```python
from build123d import *

# Parameters (mm, degrees)
F0_W      = 16
F0_H      = 16
F1_DEPTH  = 16
F2_R      = 2
F3_R      = 1.75
F4_DEPTH  = 1
F8_R      = 1.75
F8_R_2    = 1.7502183246
F9_DEPTH  = 1
F11_R     = 1.75
F12_DEPTH = 1
F14_R     = 1.75
F15_DEPTH = 1
F17_R     = 1.75
F18_DEPTH = 1
F20_R     = 1.75
F21_DEPTH = 1


# Not quite as in the source:
# - a fillet or chamfer that OpenCascade refuses, or shapes differently, is made with other operations: its cross-section is extruded or revolved along the edge and cut away or added


with BuildPart() as f1:
    # F0 (on Top) → F1 (new body)
    with BuildSketch(Plane.XY):
        Rectangle(F0_W, F0_H)
    extrude(amount=-F1_DEPTH)

    # F2
    f2_edges = [f1.edges().sort_by_distance(p)[0] for p in [
        (0, -8, 0),
        (-8, 0, 0),
        (0, 8, 0),
        (8, 0, 0),
        (8, -8, -8),
        (8, 8, -8),
        (8, 0, -16),
        (0, 8, -16),
        (-8, 8, -8),
        (-8, 0, -16),
        (-8, -8, -8),
        (0, -8, -16),
    ]]
    fillet(f2_edges, radius=F2_R)

    # F3 (on face) → F4 (cut)
    with BuildSketch(Plane.XY):
        Circle(F3_R)
        with Locations((3.89, -3.8881743788)):
            Circle(F3_R)
        with Locations((-3.89, 3.8881743788)):
            Circle(F3_R)
    extrude(amount=-F4_DEPTH, mode=Mode.SUBTRACT)

    # F5: fillet of radius 2.016187672 on 1 edges, made by hand

    # F5_s1 → F5_t2 (revolve)
    with BuildSketch(Plane.XZ.offset(3.8881743788)):
        with BuildLine():
            ThreePointArc((5.64, 0), (4.9026670776, -0.7322169988), (3.8986283154, -1))
            Line((3.8986283154, -1), (5.64, -1))
            Line((5.64, -1), (5.64, 0))
        make_face()
    revolve(axis=Axis((3.89, -3.8881743788, -1), (0, 0, 1)))

    # F6: fillet of radius 2.016187672 on 1 edges, made by hand

    # F6_s1 → F6_t2 (revolve)
    with BuildSketch(Plane.XZ):
        with BuildLine():
            ThreePointArc((1.75, 0), (1.0126670776, -0.7322169988), (0.0086283154, -1))
            Line((0.0086283154, -1), (1.75, -1))
            Line((1.75, -1), (1.75, 0))
        make_face()
    revolve(axis=Axis((0, 0, -1), (0, 0, 1)))

    # F7: fillet of radius 2.016187672 on 1 edges, made by hand

    # F7_s1 → F7_t2 (revolve)
    with BuildSketch(Plane.XZ.offset(-3.8881743788)):
        with BuildLine():
            ThreePointArc((-2.14, 0), (-2.8773329224, -0.7322169988), (-3.8813716846, -1))
            Line((-3.8813716846, -1), (-2.14, -1))
            Line((-2.14, -1), (-2.14, 0))
        make_face()
    revolve(axis=Axis((-3.89, 3.8881743788, -1), (0, 0, 1)))

    # F8 (on face) → F9 (cut)
    with BuildSketch(Plane(origin=(0, 0, -16), x_dir=(1, 0, 0), z_dir=(0, 0, -1))):
        with Locations((-3.8887145573, 3.88946)):
            Circle(F8_R)
        with Locations((3.88946, 3.8887145573)):
            Circle(F8_R)
        with Locations((-3.8892416754, -3.8892416754)):
            Circle(F8_R_2)
        with Locations((3.8892416754, -3.8892416754)):
            Circle(F8_R_2)
    extrude(amount=-F9_DEPTH, mode=Mode.SUBTRACT)

    # F10: fillet of radius 2.016187672 on 4 edges, made by hand

    # F10_s1 → F10_t2 (revolve)
    with BuildSketch(Plane.XZ.offset(3.88946)):
        with BuildLine():
            ThreePointArc((-2.1387145573, -16), (-2.8760474797, -15.2677830012), (-3.8800862419, -15))
            Line((-3.8800862419, -15), (-2.1387145573, -15))
            Line((-2.1387145573, -15), (-2.1387145573, -16))
        make_face()
    revolve(axis=Axis((-3.8887145573, -3.88946, -15), (0, 0, -1)))

    # F10_s3 → F10_t4 (revolve)
    with BuildSketch(Plane.XZ.offset(3.8887145573)):
        with BuildLine():
            ThreePointArc((5.63946, -16), (4.9021270776, -15.2677830012), (3.8980883154, -15))
            Line((3.8980883154, -15), (5.63946, -15))
            Line((5.63946, -15), (5.63946, -16))
        make_face()
    revolve(axis=Axis((3.88946, -3.8887145573, -15), (0, 0, -1)))

    # F10_s5 → F10_t6 (revolve)
    with BuildSketch(Plane.XZ.offset(-3.8892416754)):
        with BuildLine():
            ThreePointArc((-2.1390233507, -16), (-2.8763562731, -15.2677830012), (-3.8803950353, -15))
            Line((-3.8803950353, -15), (-2.1390233507, -15))
            Line((-2.1390233507, -15), (-2.1390233507, -16))
        make_face()
    revolve(axis=Axis((-3.8892416754, 3.8892416754, -15), (0, 0, -1)))

    # F10_s7 → F10_t8 (revolve)
    with BuildSketch(Plane.XZ.offset(-3.8892416754)):
        with BuildLine():
            ThreePointArc((5.63946, -16), (4.9021270776, -15.2677830012), (3.8980883154, -15))
            Line((3.8980883154, -15), (5.63946, -15))
            Line((5.63946, -15), (5.63946, -16))
        make_face()
    revolve(axis=Axis((3.8892416754, 3.8892416754, -15), (0, 0, -1)))

    # F11 (on face) → F12 (cut)
    with BuildSketch(Plane(origin=(0, 8, 0), x_dir=(-1, 0, 0), z_dir=(0, 1, 0))):
        with Locations((0, -8)):
            Circle(F11_R)
        with Locations((-3.88946, -4.11)):
            Circle(F11_R)
        with Locations((-3.88946, -11.88946)):
            Circle(F11_R)
        with Locations((3.88946, -11.88946)):
            Circle(F11_R)
        with Locations((3.88946, -4.11054)):
            Circle(F11_R)
    extrude(amount=-F12_DEPTH, mode=Mode.SUBTRACT)

    # F13: fillet of radius 2.016187672 on 5 edges, made by hand

    # F13_s1 → F13_t2 (revolve)
    with BuildSketch(Plane.XY.offset(-4.11)):
        with BuildLine():
            ThreePointArc((2.13946, 8), (2.8767929224, 7.2677830012), (3.8808316846, 7))
            Line((3.8808316846, 7), (2.13946, 7))
            Line((2.13946, 7), (2.13946, 8))
        make_face()
    revolve(axis=Axis((3.88946, 7, -4.11), (0, 1, 0)))

    # F13_s3 → F13_t4 (revolve)
    with BuildSketch(Plane.XY.offset(-8)):
        with BuildLine():
            ThreePointArc((-1.75, 8), (-1.0126670776, 7.2677830012), (-0.0086283154, 7))
            Line((-0.0086283154, 7), (-1.75, 7))
            Line((-1.75, 7), (-1.75, 8))
        make_face()
    revolve(axis=Axis((0, 7, -8), (0, 1, 0)))

    # F13_s5 → F13_t6 (revolve)
    with BuildSketch(Plane.XY.offset(-11.88946)):
        with BuildLine():
            ThreePointArc((2.13946, 8), (2.8767929224, 7.2677830012), (3.8808316846, 7))
            Line((3.8808316846, 7), (2.13946, 7))
            Line((2.13946, 7), (2.13946, 8))
        make_face()
    revolve(axis=Axis((3.88946, 7, -11.88946), (0, 1, 0)))

    # F13_s7 → F13_t8 (revolve)
    with BuildSketch(Plane.XY.offset(-11.88946)):
        with BuildLine():
            ThreePointArc((-5.63946, 8), (-4.9021270776, 7.2677830012), (-3.8980883154, 7))
            Line((-3.8980883154, 7), (-5.63946, 7))
            Line((-5.63946, 7), (-5.63946, 8))
        make_face()
    revolve(axis=Axis((-3.88946, 7, -11.88946), (0, 1, 0)))

    # F13_s9 → F13_t10 (revolve)
    with BuildSketch(Plane.XY.offset(-4.11054)):
        with BuildLine():
            ThreePointArc((-5.63946, 8), (-4.9021270776, 7.2677830012), (-3.8980883154, 7))
            Line((-3.8980883154, 7), (-5.63946, 7))
            Line((-5.63946, 7), (-5.63946, 8))
        make_face()
    revolve(axis=Axis((-3.88946, 7, -4.11054), (0, 1, 0)))

    # F14 (on face) → F15 (cut)
    with BuildSketch(Plane.YZ.offset(8)):
        with Locations((3.89, -4.11)):
            Circle(F14_R)
        with Locations((3.89, -8)):
            Circle(F14_R)
        with Locations((3.89, -11.89)):
            Circle(F14_R)
        with Locations((-3.89, -8)):
            Circle(F14_R)
        with Locations((-3.89, -4.11)):
            Circle(F14_R)
        with Locations((-3.89, -11.89)):
            Circle(F14_R)
    extrude(amount=-F15_DEPTH, mode=Mode.SUBTRACT)

    # F16: fillet of radius 2.016187672 on 6 edges, made by hand

    # F16_s1 → F16_t2 (revolve)
    with BuildSketch(Plane.XY.offset(-11.89)):
        with BuildLine():
            ThreePointArc((8, -2.14), (7.2677830012, -2.8773329224), (7, -3.8813716846))
            Line((7, -3.8813716846), (7, -2.14))
            Line((7, -2.14), (8, -2.14))
        make_face()
    revolve(axis=Axis((7, -3.89, -11.89), (1, 0, 0)))

    # F16_s3 → F16_t4 (revolve)
    with BuildSketch(Plane.XY.offset(-8)):
        with BuildLine():
            ThreePointArc((8, -2.14), (7.2677830012, -2.8773329224), (7, -3.8813716846))
            Line((7, -3.8813716846), (7, -2.14))
            Line((7, -2.14), (8, -2.14))
        make_face()
    revolve(axis=Axis((7, -3.89, -8), (1, 0, 0)))

    # F16_s5 → F16_t6 (revolve)
    with BuildSketch(Plane.XY.offset(-4.11)):
        with BuildLine():
            ThreePointArc((8, -2.14), (7.2677830012, -2.8773329224), (7, -3.8813716846))
            Line((7, -3.8813716846), (7, -2.14))
            Line((7, -2.14), (8, -2.14))
        make_face()
    revolve(axis=Axis((7, -3.89, -4.11), (1, 0, 0)))

    # F16_s7 → F16_t8 (revolve)
    with BuildSketch(Plane.XY.offset(-8)):
        with BuildLine():
            ThreePointArc((8, 5.64), (7.2677830012, 4.9026670776), (7, 3.8986283154))
            Line((7, 3.8986283154), (7, 5.64))
            Line((7, 5.64), (8, 5.64))
        make_face()
    revolve(axis=Axis((7, 3.89, -8), (1, 0, 0)))

    # F16_s9 → F16_t10 (revolve)
    with BuildSketch(Plane.XY.offset(-11.89)):
        with BuildLine():
            ThreePointArc((8, 5.64), (7.2677830012, 4.9026670776), (7, 3.8986283154))
            Line((7, 3.8986283154), (7, 5.64))
            Line((7, 5.64), (8, 5.64))
        make_face()
    revolve(axis=Axis((7, 3.89, -11.89), (1, 0, 0)))

    # F16_s11 → F16_t12 (revolve)
    with BuildSketch(Plane.XY.offset(-4.11)):
        with BuildLine():
            ThreePointArc((8, 5.64), (7.2677830012, 4.9026670776), (7, 3.8986283154))
            Line((7, 3.8986283154), (7, 5.64))
            Line((7, 5.64), (8, 5.64))
        make_face()
    revolve(axis=Axis((7, 3.89, -4.11), (1, 0, 0)))

    # F17 (on face) → F18 (cut)
    with BuildSketch(Plane(origin=(-8, 0, 0), x_dir=(0, -1, 0), z_dir=(-1, 0, 0))):
        with Locations((0, -8)):
            Circle(F17_R)
    extrude(amount=-F18_DEPTH, mode=Mode.SUBTRACT)

    # F19: fillet of radius 2.016187672 on 1 edges, made by hand

    # F19_s1 → F19_t2 (revolve)
    with BuildSketch(Plane.XY.offset(-8)):
        with BuildLine():
            ThreePointArc((-8, -1.75), (-7.2677830012, -1.0126670776), (-7, -0.0086283154))
            Line((-7, -0.0086283154), (-7, -1.75))
            Line((-7, -1.75), (-8, -1.75))
        make_face()
    revolve(axis=Axis((-7, 0, -8), (-1, 0, 0)))

    # F20 (on face) → F21 (cut)
    with BuildSketch(Plane.XZ.offset(8)):
        with Locations((-3.89, -11.89)):
            Circle(F20_R)
        with Locations((3.89, -4.11)):
            Circle(F20_R)
    extrude(amount=-F21_DEPTH, mode=Mode.SUBTRACT)

    # F22: fillet of radius 2.016187672 on 2 edges, made by hand

    # F22_s1 → F22_t2 (revolve)
    with BuildSketch(Plane.XY.offset(-11.89)):
        with BuildLine():
            ThreePointArc((-2.14, -8), (-2.8773329224, -7.2677830012), (-3.8813716846, -7))
            Line((-3.8813716846, -7), (-2.14, -7))
            Line((-2.14, -7), (-2.14, -8))
        make_face()
    revolve(axis=Axis((-3.89, -7, -11.89), (0, -1, 0)))

    # F22_s3 → F22_t4 (revolve)
    with BuildSketch(Plane.XY.offset(-4.11)):
        with BuildLine():
            ThreePointArc((5.64, -8), (4.9026670776, -7.2677830012), (3.8986283154, -7))
            Line((3.8986283154, -7), (5.64, -7))
            Line((5.64, -7), (5.64, -8))
        make_face()
    revolve(axis=Axis((3.89, -7, -4.11), (0, -1, 0)))


solid = f1.part
```
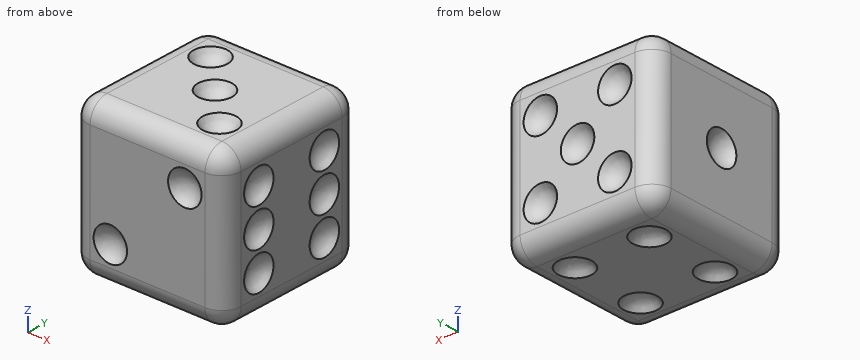
Design review of the part built by this model. Coordinates are the model's own, in mm. Give positions to 0.01 mm unless a question says otherwise; leave off trailing zeros. Order: outer loops, then holes, each group sorted by start corner. A loop starts at its lowest first (then second) coordinate and runs counter-clockwise, first axis right, second up. Notation, with made-up numbers: M -28,60 L -17,60 A10 ccw -17,66 Z; hole C 45,49 d9. An arc over 180 degrees is marked long. One line per question, with ' | ' between items. Start each with the question number.
Q1. We need section B-B (y = -6.5). Write out the cut boundary in (x, z), plus the area to 3 significant figures.
Q2. For L1, parallel to Y at x = -0.25, z = -9.25; L2, parallel to X at y = 3.75, z = -10.5; L3, parallel to Z at x = -7.25, y = -2.5, list the stretches that pass through material, from the lowest coordinate up. Write a range as [from, to].
Q3. We need section A-A (z = -14.5). Write out the cut boundary in (x, y), plus the area to 3 significant figures.
Returned:
1) outline: M -7.94,-14 A1.94 ccw -6,-15.94 L 6,-15.94 A1.94 ccw 7.94,-14 L 7.94,-2 A1.94 ccw 6,-0.06 L -6,-0.06 A1.94 ccw -7.94,-2 Z | area: 249 mm2
2) L1: [-8, 7.45] | L2: [-8, 7.55] | L3: [-15.56, -0.44]
3) outline: M -7.94,-6 A1.94 ccw -6,-7.94 L 6,-7.94 A1.94 ccw 7.94,-6 L 7.94,6 A1.94 ccw 6,7.94 L -6,7.94 A1.94 ccw -7.94,6 Z | area: 249 mm2
